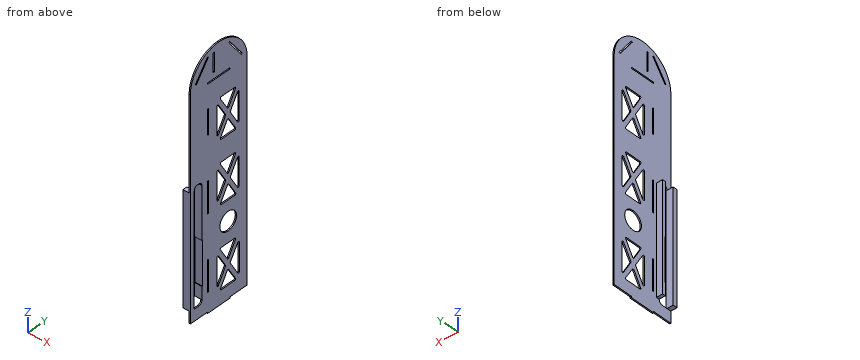
from build123d import *

# Parameters (mm, degrees)
SKETCH_1_W      = 40
SKETCH_1_H      = 2
SKETCH_1_W_2    = 50
SKETCH_1_R      = 15
SKETCH_1_W_3    = 30
SKETCH_1_W_4    = 2
SKETCH_1_H_2    = 40
EXTRUDE_3_DEPTH = 2
SKETCH_2_W      = 180.5
SKETCH_2_H      = 7
EXTRUDE_4_DEPTH = 12


with BuildPart() as part:
    # 草图1 → 凸台-拉伸3 (new body)
    # profile 1 of 4: a face of its own
    with BuildSketch(Plane(origin=(0, 0, 0), x_dir=(0, 0, -1), z_dir=(1, 0, 0))):
        Polygon((139, 51), (0, 51), (0, 20), (2, 20), (2, -20), (0, -20), (0, -51), (350, -51), (350, -20), (350, 20), (350, 51), (337.5, 51), (331.5, 51), (145, 51), align=None)
        with Locations((59.999999544, -18.999999639)):
            Rectangle(SKETCH_1_W, SKETCH_1_H, mode=Mode.SUBTRACT)
        with BuildLine():
            Line((145, -38), (145, -36))
            ThreePointArc((145, -36), (146.757359313, -31.757359313), (151, -30))
            Line((151, -30), (235, -30))
            Line((235, -30), (235, -29.2))
            Line((235, -29.2), (305, -29.2))
            Line((305, -29.2), (305, -30))
            Line((305, -30), (325.5, -30))
            ThreePointArc((325.5, -30), (329.742640687, -31.757359313), (331.5, -36))
            Line((331.5, -36), (331.5, -39))
            Line((331.5, -39), (331.5, -44))
            Line((331.5, -44), (325.5, -44))
            Line((325.5, -44), (151, -44))
            ThreePointArc((151, -44), (146.757359313, -42.242640687), (145, -38))
        make_face(mode=Mode.SUBTRACT)
        with Locations((174.999999544, -18.999999639)):
            Rectangle(SKETCH_1_W_2, SKETCH_1_H, mode=Mode.SUBTRACT)
        with Locations((294.999999544, -18.999999639)):
            Rectangle(SKETCH_1_W_2, SKETCH_1_H, mode=Mode.SUBTRACT)
        with BuildLine():
            Line((35.191745107, 4.260800891), (35.191745107, 29.047933032))
            ThreePointArc((35.191745107, 29.047933032), (35.944654017, 30.348646261), (37.447551645, 30.343601384))
            Line((37.447551645, 30.343601384), (58.776761499, 17.901562302))
            ThreePointArc((58.776761499, 17.901562302), (59.520952796, 16.603345479), (58.772354511, 15.307664881))
            Line((58.772354511, 15.307664881), (37.443144656, 2.962571821))
            ThreePointArc((37.443144656, 2.962571821), (35.942445208, 2.961358833), (35.191745107, 4.260800891))
        make_face(mode=Mode.SUBTRACT)
        with BuildLine():
            Line((89.643364252, -3.340511469), (45.740125962, -3.340511469))
            ThreePointArc((45.740125962, -3.340511469), (44.292109641, -2.231981438), (44.984319423, -0.544843118))
            Line((44.984319423, -0.544843118), (66.935938568, 12.26026805))
            ThreePointArc((66.935938568, 12.26026805), (67.691745107, 12.464599699), (68.447551645, 12.26026805))
            Line((68.447551645, 12.26026805), (90.39917079, -0.544843118))
            ThreePointArc((90.39917079, -0.544843118), (91.091380572, -2.231981438), (89.643364252, -3.340511469))
        make_face(mode=Mode.SUBTRACT)
        with BuildLine():
            ThreePointArc((97.935938568, 30.343601384), (99.438836196, 30.348646261), (100.191745107, 29.047933032))
            Line((100.191745107, 29.047933032), (100.191745107, 4.27104403))
            ThreePointArc((100.191745107, 4.27104403), (99.438836196, 2.970330801), (97.935938568, 2.975375678))
            Line((97.935938568, 2.975375678), (76.698605138, 15.36382018))
            ThreePointArc((76.698605138, 15.36382018), (75.954411676, 16.659488531), (76.698605138, 17.955156882))
            Line((76.698605138, 17.955156882), (97.935938568, 30.343601384))
        make_face(mode=Mode.SUBTRACT)
        with BuildLine():
            Line((134.999999544, 4.260800891), (134.999999544, 29.047933032))
            ThreePointArc((134.999999544, 29.047933032), (135.752908454, 30.348646261), (137.255806082, 30.343601384))
            Line((137.255806082, 30.343601384), (158.585015936, 17.901562302))
            ThreePointArc((158.585015936, 17.901562302), (159.329207233, 16.603345479), (158.580608948, 15.307664881))
            Line((158.580608948, 15.307664881), (137.251399093, 2.962571821))
            ThreePointArc((137.251399093, 2.962571821), (135.750699645, 2.961358833), (134.999999544, 4.260800891))
        make_face(mode=Mode.SUBTRACT)
        with BuildLine():
            ThreePointArc((44.984319423, 33.86382018), (44.292109641, 35.5509585), (45.740125962, 36.659488531))
            Line((45.740125962, 36.659488531), (90.076890905, 36.659488531))
            ThreePointArc((90.076890905, 36.659488531), (91.525570236, 35.548497783), (90.828290455, 33.861259462))
            Line((90.828290455, 33.861259462), (68.573204266, 20.980280188))
            ThreePointArc((68.573204266, 20.980280188), (67.819256245, 20.778511422), (67.065998178, 20.982840906))
            Line((67.065998178, 20.982840906), (44.984319423, 33.86382018))
        make_face(mode=Mode.SUBTRACT)
        with BuildLine():
            Line((189.451618689, -3.340511469), (145.548380399, -3.340511469))
            ThreePointArc((145.548380399, -3.340511469), (144.100364078, -2.231981438), (144.79257386, -0.544843118))
            Line((144.79257386, -0.544843118), (166.744193005, 12.26026805))
            ThreePointArc((166.744193005, 12.26026805), (167.499999544, 12.464599699), (168.255806082, 12.26026805))
            Line((168.255806082, 12.26026805), (190.207425227, -0.544843118))
            ThreePointArc((190.207425227, -0.544843118), (190.899635009, -2.231981438), (189.451618689, -3.340511469))
        make_face(mode=Mode.SUBTRACT)
        with BuildLine():
            ThreePointArc((197.744193005, 30.684113214), (199.247090633, 30.689158091), (199.999999544, 29.388444862))
            Line((199.999999544, 29.388444862), (199.999999544, 4.61155586))
            ThreePointArc((199.999999544, 4.61155586), (199.247090633, 3.310842631), (197.744193005, 3.315887508))
            Line((197.744193005, 3.315887508), (176.506859575, 15.70433201))
            ThreePointArc((176.506859575, 15.70433201), (175.762666113, 17.000000361), (176.506859575, 18.295668712))
            Line((176.506859575, 18.295668712), (197.744193005, 30.684113214))
        make_face(mode=Mode.SUBTRACT)
        with Locations((232.499999544, 17.000000361)):
            Circle(SKETCH_1_R, mode=Mode.SUBTRACT)
        with BuildLine():
            Line((319.974166341, -3.394327578), (276.070928051, -3.394327578))
            ThreePointArc((276.070928051, -3.394327578), (274.622911731, -2.285797546), (275.315121513, -0.598659226))
            Line((275.315121513, -0.598659226), (297.266740658, 12.206451942))
            ThreePointArc((297.266740658, 12.206451942), (298.022547196, 12.41078359), (298.778353734, 12.206451942))
            Line((298.778353734, 12.206451942), (320.729972879, -0.598659226))
            ThreePointArc((320.729972879, -0.598659226), (321.422182661, -2.285797546), (319.974166341, -3.394327578))
        make_face(mode=Mode.SUBTRACT)
        with BuildLine():
            Line((265.522547196, 4.206984782), (265.522547196, 28.994116924))
            ThreePointArc((265.522547196, 28.994116924), (266.275456106, 30.294830153), (267.778353734, 30.289785275))
            Line((267.778353734, 30.289785275), (289.107563589, 17.847746193))
            ThreePointArc((289.107563589, 17.847746193), (289.851754885, 16.549529371), (289.1031566, 15.253848773))
            Line((289.1031566, 15.253848773), (267.773946745, 2.908755713))
            ThreePointArc((267.773946745, 2.908755713), (266.273247297, 2.907542724), (265.522547196, 4.206984782))
        make_face(mode=Mode.SUBTRACT)
        with BuildLine():
            ThreePointArc((327.730104048, 30.281463391), (329.239984934, 30.298885724), (329.999999544, 28.994116924))
            Line((329.999999544, 28.994116924), (329.999999544, 4.522047385))
            ThreePointArc((329.999999544, 4.522047385), (329.247090633, 3.221334156), (327.744193005, 3.226379034))
            Line((327.744193005, 3.226379034), (307.029407227, 15.310004071))
            ThreePointArc((307.029407227, 15.310004071), (306.285236078, 16.597490851), (307.01531827, 17.893018889))
            Line((307.01531827, 17.893018889), (327.730104048, 30.281463391))
        make_face(mode=Mode.SUBTRACT)
        with BuildLine():
            ThreePointArc((144.79257386, 33.86382018), (144.100364078, 35.5509585), (145.548380399, 36.659488531))
            Line((145.548380399, 36.659488531), (189.885145343, 36.659488531))
            ThreePointArc((189.885145343, 36.659488531), (191.333824673, 35.548497783), (190.636544892, 33.861259462))
            Line((190.636544892, 33.861259462), (168.381458703, 20.980280188))
            ThreePointArc((168.381458703, 20.980280188), (167.627510682, 20.778511422), (166.874252615, 20.982840906))
            Line((166.874252615, 20.982840906), (144.79257386, 33.86382018))
        make_face(mode=Mode.SUBTRACT)
        with BuildLine():
            ThreePointArc((275.298058871, 34.214436971), (274.625531032, 35.901033349), (276.070928051, 37.000000361))
            Line((276.070928051, 37.000000361), (321.088992302, 37.000000361))
            ThreePointArc((321.088992302, 37.000000361), (322.537671633, 35.889009613), (321.840391852, 34.201771291))
            Line((321.840391852, 34.201771291), (298.904006355, 20.926464079))
            ThreePointArc((298.904006355, 20.926464079), (298.140143214, 20.72474493), (297.379737626, 20.939129758))
            Line((297.379737626, 20.939129758), (275.298058871, 34.214436971))
        make_face(mode=Mode.SUBTRACT)
    # profile 2 of 4: a face of its own
    with BuildSketch(Plane(origin=(0, 0, 0), x_dir=(0, 0, -1), z_dir=(1, 0, 0))):
        with BuildLine():
            Line((0, 20), (0, 51))
            ThreePointArc((0, 51), (-36.062445841, 36.062445841), (-51, 0))
            Line((-51, 0), (0, 0))
            Line((0, 0), (0, 20))
        make_face()
        Polygon((-38.821768829, 18.383902445), (-40, 20), (-9.698170842, 42.091834457), (-8.519939671, 40.475736902), align=None, mode=Mode.SUBTRACT)
    # profile 3 of 4: a face of its own
    with BuildSketch(Plane(origin=(0, 0, 0), x_dir=(0, 0, -1), z_dir=(1, 0, 0))):
        with BuildLine():
            Line((0, 0), (-51, 0))
            ThreePointArc((-51, 0), (-36.062445841, -36.062445841), (0, -51))
            Line((0, -51), (0, -20))
            Line((0, -20), (0, 0))
        make_face()
        Polygon((-40, -20), (-38.821768829, -18.383902445), (-8.519939671, -40.475736902), (-9.698170842, -42.091834457), align=None, mode=Mode.SUBTRACT)
        with Locations((-25, -9)):
            Rectangle(SKETCH_1_W_3, SKETCH_1_H, mode=Mode.SUBTRACT)
    # profile 4 of 4: a face of its own
    with BuildSketch(Plane(origin=(0, 0, 0), x_dir=(0, 0, -1), z_dir=(1, 0, 0))):
        with Locations((351, 0)):
            Rectangle(SKETCH_1_W_4, SKETCH_1_H_2)
    extrude(amount=EXTRUDE_3_DEPTH)

    # 草图2 → 凸台-拉伸4 (add)
    with BuildSketch(Plane(origin=(2, 0, 0), x_dir=(0, 0, -1), z_dir=(1, 0, 0))):
        with Locations((241.25, -47.5)):
            Rectangle(SKETCH_2_W, SKETCH_2_H)
        Polygon((151, -30), (235, -30), (235, -29.2), (305, -29.2), (305, -30), (325.5, -30), (325.5, -25), (151, -25), align=None)
    extrude(amount=-EXTRUDE_4_DEPTH)


solid = part.part
Can you work these out from the model? Positions are in its coordinate system, mm. Give positions to 0.01 mm unless a question says otherwise; leave off trailing zeros. Loops run counter-clockwise (first coordinate to the right, second up) from the corner with the lowest first, then second, coordinate; pieces in that order, holes last. Notation, with made-up numbers: (18, 47) - (42, 47) arc R19 ccw to (42, 58) - close; hole circle Ø11 at (35, 67). An arc over 180 degrees is marked (long way). Answer as a JSON object with one key per item and string values.
Q1. Will these pins go through, and if not, where does the flat tip stop? P1, Ø1.6, axis at x = 0.5, y = 19, coming from the +Z side; P2, Ø1.6, axis at x = 1, y = -8.5, coming from the +Z side; P3, Ø18, axis at y = 17, z = -232.5, coming from the +X side; P4, Ø5.5, axis at x = -5.5, y = -27, coming from the +Z side.
Geometry says:
{"P1": "z = 47.64", "P2": "z = 50.42", "P3": "through", "P4": "z = -151"}
Q2. Imagine slicing it at D-D on z = -23. Write out the boundary of the cut face in (x, y).
Geometry says:
{"outline": "(0, -51) - (2, -51) - (2, 51) - (0, 51) - close"}
Q3. Imagine slicing it at C-C on z = -210. Write out the boundary of the cut face in (x, y).
Geometry says:
{"outline": "(-10, -51) - (2, -51) - (2, -44) - (-10, -44) - close; (-10, -30) - (2, -30) - (2, 51) - (0, 51) - (0, -25) - (-10, -25) - close"}
Q4. Imagine slicing it at B-B on x = -2. Write out the boundary of the cut face in (y, z).
Geometry says:
{"outline": "(-51, -331.5) - (-44, -331.5) - (-44, -151) - (-51, -151) - close; (-30, -325.5) - (-25, -325.5) - (-25, -151) - (-30, -151) - (-30, -235) - (-29.2, -235) - (-29.2, -305) - (-30, -305) - close"}
Q5. If I drill on L1, parallel to Y at x = 1.35, z = -232.5; L2, parallel to Y at x = -7, z = -220; L3, parallel to X at y = 21.5, z = 6, over which ranges is the centre line in solid material (lowest first)?
Geometry says:
{"L1": "-51 to -44, -30 to 2, 32 to 51", "L2": "-51 to -44, -30 to -25", "L3": "0 to 2"}
Q6. Imagine slicing it at A-A on z = -254. Write out the boundary of the cut face in (x, y), plus the area to 3 significant figures.
Geometry says:
{"outline": "(-10, -51) - (2, -51) - (2, -44) - (-10, -44) - close; (-10, -29.2) - (2, -29.2) - (2, 51) - (0, 51) - (0, -25) - (-10, -25) - close", "area": "286 mm²"}
